Geometry: final body of the model. Coordinates: model frame, mm. A direction names the side the tool comes from. Give positions to 0.01 mm unless a question says otherwise; leave off trailing zeros. Write each loop counter-clockwise with the first axis right and the second up, starting at its lowest first coordinate (ties: lowest second). Pieces come first, ordered by that corner, then holes. Notation, with made-up numbers: (25.25, 37) - (38.25, 37) arc R25 ccw to (38.25, 68) - close; hole circle Ø7 at (89.25, 31.25). An arc over 180 degrees is marked (long way). One line per question, with ' | ' between items. Start each with the question number.
Autodesk Inventor part; units mm, degrees
ref_plane "YZ Plane" through (0, 0, 0) normal (1, 0, 0) x (0, 1, 0)
ref_plane "XZ Plane" through (0, 0, 0) normal (0, 1, 0) x (-1, 0, 0)
ref_plane "XY Plane" through (0, 0, 0) normal (0, 0, 1) x (1, 0, 0)
sketch "Sketch1" plane through (0, 0, 0) normal (0, 0, 1) x (1, 0, 0)
  line L0 (-30.5, -30.5) -> (30.5, -30.5) construction
  line L1 (30.5, -30.5) -> (30.5, 30.5) construction
  line L2 (30.5, 30.5) -> (-30.5, 30.5) construction
  line L3 (-30.5, 30.5) -> (-30.5, -30.5) construction
  line L4 (-30.5, -30.5) -> (30.5, 30.5) construction
  line L5 (30.5, -30.5) -> (-30.5, 30.5) construction
  circle A0 centre (0, 0) radius 5
  circle A1 centre (-30.5, 30.5) radius 1.5
  circle A2 centre (30.5, 30.5) radius 1.5
  circle A3 centre (-30.5, -30.5) radius 1.5
  circle A4 centre (30.5, -30.5) radius 1.5
  line L6 (31.5, -32.5) -> (-31.5, -32.5)
  line L7 (-32.5, -31.5) -> (-32.5, 31.5)
  line L8 (-31.5, 32.5) -> (31.5, 32.5)
  line L9 (32.5, 31.5) -> (32.5, -31.5)
  line L10 (32.5, -32.5) -> (-32.5, 32.5) construction
  line L11 (-32.5, -32.5) -> (32.5, 32.5) construction
  arc A5 (-31.5, 32.5) -> (-32.5, 31.5) centre (-31.5, 31.5) ccw
  arc A6 (32.5, 31.5) -> (31.5, 32.5) centre (31.5, 31.5) ccw
  arc A7 (31.5, -32.5) -> (32.5, -31.5) centre (31.5, -31.5) ccw
  arc A8 (-32.5, -31.5) -> (-31.5, -32.5) centre (-31.5, -31.5) ccw
  circle A9 centre (0, 0) radius 8.75
  dimension "d0" = 61
  dimension "d1" = 61
  dimension "d2" = 10
  dimension "d3" = 3
  dimension "d4" = 3
  dimension "d5" = 3
  dimension "d6" = 3
  dimension "d7" = 0
  dimension "d8" = 61
  dimension "d9" = 65
  dimension "d10" = 65
  dimension "d11" = 1
  dimension "d12" = 17.5
extrude "Extrusion1" add sketch "Sketch1" along normal blind 7.5 contours L6 A8 L7 A5 L8 A6 L9 A7
extrude "Extrusion2" add sketch "Sketch1" along normal blind 15 contours A9
sketch "Sketch2" plane through (0, 0, 7.5) normal (0, 0, 1) x (1, 0, 0)
  line L0 (-15.5, -12.5) -> (17.5, -12.5)
  line L1 (17.5, -12.5) -> (17.5, -25.5)
  line L2 (15.5, -27.5) -> (-17.5, -27.5)
  line L3 (-17.5, -27.5) -> (-17.5, -14.5)
  line L4 (-32.5, 31.5) -> (-32.5, -31.5)
  line L5 (32.5, -31.5) -> (32.5, 31.5)
  line L6 (-31.5, -32.5) -> (31.5, -32.5)
  arc A0 (-15.5, -12.5) -> (-17.5, -14.5) centre (-15.5, -14.5) ccw
  arc A1 (15.5, -27.5) -> (17.5, -25.5) centre (15.5, -25.5) ccw
  point P0 (0, 0)
  dimension "d17" = 15
  dimension "d18" = 15
  dimension "d19" = 5
  dimension "d20" = 15
  dimension "d21" = 2
extrude "Extrusion3" cut sketch "Sketch2" against normal up to surface (7.5 mm away)
properties part number "top"
1) Line query: L1, parallel to Y at x = -30.5, z = 3.5; L2, parallel to Z at x = -18, y = -7; L3, parallel to X at y = -2.5, z = 6.25. Output: solid intervals per line, ascending.
2) Section A-A, the plane y = 0. Output: boundary loops of the cut face in (x, z).
3) Pull-direction query (Y, two-part tool) for faces 1 (the flat face through (0, -32.5, 4)), 2 (the cylindrical face through (-31.61, 29.49, 3.7)), 3 (the flat face through (0, 8, 0)), 4 (the cylindrical face through (-6.944, 5.324, 11.198)); classes: +Y half, -Y half, draft (parallel to the pull), parting line (faces both ways), or undercut.
4) Section C-C, the plane x = 0. Output: boundary loops of the cut face in (y, z).
5) Reachability of faces 5 (the cylindrical face through (-16.9, -13.07, 3.8)), 6 (the flat face through (0, 32.5, 4)) from +Z, -Z, +X, -X, +Y, -Y: full face, straight path, thin tool, end or side. Return the list, or none.
6) Section D-D, the plane y = -30.5. Output: boundary loops of the cut face in (x, z).
7) Section B-B, the plane x = -9.5. Output: boundary loops of the cut face in (y, z).
8) First-contact query: pin 1 Ø3.5 at (x, y) = (-30.5, 30.5) entering from -Z; pin 2 Ø5 at (x, y) = (23.5, 25.5) entering from +Z. Flat tips, straight axial feed; report the tip coordinate or a pass-through.
Answer key:
1) L1: -32.5 to -32, -29 to 29, 32 to 32.5 | L2: 0 to 7.5 | L3: -32.5 to -4.33, 4.33 to 32.5
2) outline: (-32.5, 0) - (-5, 0) - (-5, 15) - (-8.75, 15) - (-8.75, 7.5) - (-32.5, 7.5) - close; (5, 0) - (32.5, 0) - (32.5, 7.5) - (8.75, 7.5) - (8.75, 15) - (5, 15) - close
3) face 1: -Y half | face 2: undercut | face 3: draft | face 4: parting line
4) outline: (-32.5, 0) - (-27.5, 0) - (-27.5, 7.5) - (-32.5, 7.5) - close; (-12.5, 0) - (-5, 0) - (-5, 15) - (-8.75, 15) - (-8.75, 7.5) - (-12.5, 7.5) - close; (5, 0) - (32.5, 0) - (32.5, 7.5) - (8.75, 7.5) - (8.75, 15) - (5, 15) - close
5) face 5: +Z, -Z | face 6: +Z, -Z, +X, -X, +Y
6) outline: (-32.5, 0) - (-32, 0) - (-32, 7.5) - (-32.5, 7.5) - close; (-29, 0) - (29, 0) - (29, 7.5) - (-29, 7.5) - close; (32, 0) - (32.5, 0) - (32.5, 7.5) - (32, 7.5) - close
7) outline: (-32.5, 0) - (-27.5, 0) - (-27.5, 7.5) - (-32.5, 7.5) - close; (-12.5, 0) - (32.5, 0) - (32.5, 7.5) - (-12.5, 7.5) - close
8) pin 1: z = 0 | pin 2: z = 7.5
